Read the model definition and answer for the solid it produces. Units are mm, in the model's axes. A direction names the side the tool comes from. Coordinates: 2 decimals unless noted, no trailing zeros. Answer as a JSON object with one key per item and string values. Group by question number.
(1) Flat-ended cylindrical pins translate along their axes: P1, Ø2, axis at x = 25, z = 129.5, coming from the +Y side; P2, Ø0.7, axis at x = 30, z = 191, coming from the -Y side; P3, Ø1.9, axis at x = 62, z = 161, coming from the +Y side. Find the tip coordinate at first contact, or state that the pin passes through.
(2) Find section A-A (y = 28). Count the separate pieces of the cut face and the enclosed holes in it, then the cut area to 3 significant figures.
(3) Which of the six approach directions +Z, -Z, +X, -X, +Y, -Y give full straight-line access (tool end or side, diameter ignored) to faces 1 (the face through (69.884, 22.984, 167.31)), 2 (the face through (61, 13, 0))?
(4) Straight lines are drawn through the part: L1, parallel to Z at x = 67, y = 2.45; L2, parallel to X at y = 3.5, z = 8; L3, parallel to Z at x = 26, y = 3. For each, find the intervals that lie inside material, in ascending order.
(5) For a pull along X with two mould halves and no side action, classify faces 3 (the face through (62, 0, 163)), 4 (the face through (0, 20, 163)), 5 (the face through (29.884, 22.984, 167.31)) as +X half, -X half, draft (parallel to the pull), parting line (faces both ways), or undercut.
from build123d import *

# Parameters (mm, degrees)
EXTRUDE_1_DEPTH       = 330
EXTRUDE_3_DEPTH       = 330
PATTERN_CURVE_1_COUNT = 11
PATTERN_CURVE_1_PITCH = 10
SKETCH_3_R            = 2.25
CUT_EXTRUDE_1_DEPTH   = 6
SKETCH_4_R            = 1.6
CUT_EXTRUDE_2_DEPTH   = 6


with BuildPart() as part:
    # Эскиз1 → Вытянуть1 (new body)
    with BuildSketch(Plane.XY):
        with BuildLine():
            Line((0, 40), (1.528979332, 40))
            ThreePointArc((1.528979332, 40), (2.225614441, 39.717425624), (2.528547087, 39.029399052))
            Line((2.528547087, 39.029399052), (3.5, 6))
            Line((3.5, 6), (118.5, 6))
            Line((118.5, 6), (119.471452913, 39.029399052))
            ThreePointArc((119.471452913, 39.029399052), (119.774385559, 39.717425624), (120.471020668, 40))
            Line((120.471020668, 40), (122, 40))
            Line((122, 40), (122, 0))
            Line((122, 0), (0, 0))
            Line((0, 0), (0, 40))
        make_face()
    extrude(amount=EXTRUDE_1_DEPTH)

    # Эскиз2 → Вытянуть3 (add)
    with BuildSketch(Plane.XY.offset(330)):
        with BuildLine():
            Line((10.5, 39.5), (9.25, 6))
            Line((9.25, 6), (12.75, 6))
            Line((12.75, 6), (11.5, 39.5))
            ThreePointArc((11.5, 39.5), (11, 40), (10.5, 39.5))
        make_face()
    extrude_3 = extrude(amount=-EXTRUDE_3_DEPTH)

    # Кривая1: Вытянуть3 ×11
    with Locations(*[(i * PATTERN_CURVE_1_PITCH, 0, 0) for i in range(1, PATTERN_CURVE_1_COUNT)]):
        add(extrude_3)

    # Эскиз3 → Вырез-Вытянуть1 (cut)
    with BuildSketch(Plane.XZ):
        with Locations((26, 322)):
            Circle(SKETCH_3_R)
        with Locations((96, 322)):
            Circle(SKETCH_3_R)
        with Locations(Location((96, 8, 0), (0, 0, 180))):
            Circle(SKETCH_3_R)
        with Locations(Location((26, 8, 0), (0, 0, 180))):
            Circle(SKETCH_3_R)
    extrude(amount=-CUT_EXTRUDE_1_DEPTH, mode=Mode.SUBTRACT)

    # Эскиз4 → Вырез-Вытянуть2 (cut)
    with BuildSketch(Plane(origin=(147.933613103, 0, 237.946321054), x_dir=(-1, 0, 0), z_dir=(0, -1, 0))):
        with Locations(Location((80.933613103, -68.053678946, 0), (0, 0, 180))):
            Circle(SKETCH_4_R)
        with Locations(Location((42.433613103, 124.346321054, 0), (0, 0, 180))):
            Circle(SKETCH_4_R)
        with Locations(Location((85.933613103, 211.946321054, 0), (0, 0, 180))):
            Circle(SKETCH_4_R)
        with Locations(Location((85.933613103, 76.946321054, 0), (0, 0, 180))):
            Circle(SKETCH_4_R)
        with Locations(Location((80.933613103, 61.946321054, 0), (0, 0, 180))):
            Circle(SKETCH_4_R)
        with Locations(Location((118.933613103, 46.446321054, 0), (0, 0, 180))):
            Circle(SKETCH_4_R)
    extrude(amount=-CUT_EXTRUDE_2_DEPTH, mode=Mode.SUBTRACT)


solid = part.part
Results below:
{
 "1": {"P1": "stops at y = 6", "P2": "stops at y = 6", "P3": "stops at y = 40"},
 "2": {"separate pieces": "13", "enclosed holes": "0", "area": "8,630 mm2"},
 "3": {"face 1": "+Z, -Z, +Y", "face 2": "-Z, +X, -X, +Y, -Y"},
 "4": {"L1": "z = 0 to 174.4, 177.6 to 304.4, 307.6 to 330", "L2": "x = 0 to 23.75, 28.25 to 93.75, 98.25 to 122", "L3": "z = 0 to 5.75, 10.25 to 319.75, 324.25 to 330"},
 "5": {"face 3": "draft", "face 4": "-X half", "face 5": "undercut"}
}
